Geometry check sheet. Reference: the model listing, model coordinates, mm. A direction names the side the tool comes from. Coordinates: 2 decimals unless noted, no trailing zeros. Write each loop counter-clockwise with the first axis right and the second up, starting at its lowest first coordinate (ties: lowest second). Pieces come first, ordered by that corner, then holes. Notation, with made-up numbers: M 68,38 L 112,38 A9 ccw 112,43 Z; hole C 67,20 d9. An arc over 180 degrees is marked long. Put each result on its own line as item: value. Start each with the question number.
1) Cross-section at B-B on z = -1.75. Count the separate pieces of the cut face and the enclosed holes in it, plus the area to 3 significant figures.
2) Cross-section at A-A on z = 2.5. Record the cut outline in (x, y).
3) Mould release check, pull along Y, two halves, no side actions. Record for faces 5 (the flat face through (-10.555, 0, 0)), 6 (the flat face through (10.555, 0, 0)), 7 (the flat face through (0, -11, -0.4)): released by +Y, released by -Y, zero draft, split by the parting line, or undercut.
4) Cross-section at C-C on y = 8.25. Record the cut outline in (x, z), plus the area to 3 significant figures.
5) Set-up check for faces 1 (the flat face through (-2.65, -10, -2)), 2 (the flat face through (10, 2.65, -2)), 3 (the flat face through (13.989, 0, 2)), 4 (the flat face through (1.6, -9, 1)): record each of +Z, -Z, +X, -X, +Y, -Y from which the full face is reachable in a straight line by a thin tool's end or side.
6) Scan lines: line 1 along X through (y, z) = (-8.25, 1.25); line 2 along X through (y, z) = (9.75, -0.5). Record each from-to range of solid material in increasing order.
7) Gauge pin test, flat ends, axial feed: pin 1 (2 mm diameter, centred on x = -10, z = 0.5, fed in from +Y); pin 2 (1.5 mm diameter, centred on y = -9.5, z = 3.5, fed in from -X); pin 3 (2.5 mm diameter, centred on x = -10, y = 0, fed in from -Z). Record the tip position at first contact, or that the pin passes through.
from build123d import *

# Parameters (mm, degrees)
PAD001_DEPTH    = 6.5
POCKET003_DEPTH = 5.5
PAD002_DEPTH    = 3.5
FILLET007_R     = 1
PAD009_DEPTH    = 2.4
FILLET_R        = 1
FILLET009_R     = 1
SKETCH025_W     = 5.3
SKETCH025_H     = 2
SKETCH025_W_2   = 2
SKETCH025_H_2   = 5.3
POCKET005_DEPTH = 3.1


with BuildPart() as part:
    # Sketch003 → Revolution001 (revolve)
    with BuildSketch(Plane.XZ):
        with BuildLine():
            Line((6, 3), (8, 3))
            ThreePointArc((8, 3), (7.795832, 4.795832), (7.193747, 6.5))
            Line((7.193747, 6.5), (4.570714, 6.5))
            ThreePointArc((6, 3), (5.628908, 4.890295), (4.570714, 6.5))
        make_face()
    revolve(axis=Axis((0, 0, 0), (0, 0, 1)))

    # Sketch004 (on Face1 of Revolution001) → Pad001 (new body)
    with BuildSketch(Plane(origin=(0, 0, 3), x_dir=(1, 0, 0), z_dir=(0, 0, -1))):
        with BuildLine():
            Line((4.65, -5.488852), (4.65, -13.988852))
            Line((4.65, -13.988852), (-4.65, -13.988852))
            Line((-4.65, -13.988852), (-4.65, -5.488852))
            ThreePointArc((-4.65, -5.488852), (0, -7.193747), (4.65, -5.488852))
        make_face()
        with BuildLine():
            Line((-5.488852, -4.65), (-13.988852, -4.65))
            Line((-13.988852, -4.65), (-13.988852, 4.65))
            Line((-13.988852, 4.65), (-5.488852, 4.65))
            ThreePointArc((-5.488852, 4.65), (-7.193747, 0), (-5.488852, -4.65))
        make_face()
        with BuildLine():
            Line((13.988852, -4.65), (13.988852, 4.65))
            Line((5.488852, 4.65), (13.988852, 4.65))
            ThreePointArc((5.488852, -4.65), (7.193747, 0), (5.488852, 4.65))
            Line((5.488852, -4.65), (13.988852, -4.65))
        make_face()
        with BuildLine():
            Line((-4.65, 5.488852), (-4.65, 13.988852))
            Line((-4.65, 13.988852), (4.65, 13.988852))
            Line((4.65, 13.988852), (4.65, 5.488852))
            ThreePointArc((4.65, 5.488852), (0, 7.193747), (-4.65, 5.488852))
        make_face()
    extrude(amount=PAD001_DEPTH)

    # Sketch018 (on Face24 of Pad001) → Pocket003 (cut)
    with BuildSketch(Plane(origin=(0, 0, -3.5), x_dir=(1, 0, 0), z_dir=(0, 0, -1))):
        with BuildLine():
            Line((-6.687862, 2.65), (-11.988852, 2.65))
            Line((-11.988852, 2.65), (-11.988852, -2.65))
            Line((-11.988852, -2.65), (-6.687862, -2.65))
            ThreePointArc((-6.687862, 2.65), (-7.193747, 0), (-6.687862, -2.65))
        make_face()
        with BuildLine():
            Line((-2.65, 6.687862), (-2.65, 11.988852))
            Line((-2.65, 11.988852), (2.65, 11.988852))
            Line((2.65, 11.988852), (2.65, 6.687862))
            ThreePointArc((2.65, 6.687862), (0, 7.193747), (-2.65, 6.687862))
        make_face()
        with BuildLine():
            Line((6.687862, 2.65), (11.988852, 2.65))
            Line((11.988852, 2.65), (11.988852, -2.65))
            Line((11.988852, -2.65), (6.687862, -2.65))
            ThreePointArc((6.687862, -2.65), (7.193747, 0), (6.687862, 2.65))
        make_face()
        with BuildLine():
            Line((2.65, -6.687862), (2.65, -11.988852))
            Line((2.65, -11.988852), (-2.65, -11.988852))
            Line((-2.65, -11.988852), (-2.65, -6.687862))
            ThreePointArc((-2.65, -6.687862), (0, -7.193747), (2.65, -6.687862))
        make_face()
    extrude(amount=-POCKET003_DEPTH, mode=Mode.SUBTRACT)

    # Sketch006 (on Face19 of Pocket003) → Pad002 (join)
    with BuildSketch(Plane(origin=(0, 0, 3), x_dir=(-1, 0, 0), z_dir=(0, 0, 1))):
        with BuildLine():
            Line((-13.988852, 4.65), (-5.488852, 4.65))
            ThreePointArc((-5.488852, 4.65), (-7.193747, 0), (-5.488852, -4.65))
            Line((-13.988852, -4.65), (-5.488852, -4.65))
            Line((-13.988852, -4.65), (-13.988852, 4.65))
        make_face()
        with BuildLine():
            Line((-4.65, 13.988852), (-4.65, 5.488852))
            ThreePointArc((4.65, 5.488852), (0, 7.193747), (-4.65, 5.488852))
            Line((4.65, 13.988852), (4.65, 5.488852))
            Line((-4.65, 13.988852), (4.65, 13.988852))
        make_face()
        with BuildLine():
            Line((5.488852, 4.65), (13.988852, 4.65))
            Line((13.988852, 4.65), (13.988852, -4.65))
            Line((13.988852, -4.65), (5.488852, -4.65))
            ThreePointArc((5.488852, -4.65), (7.193747, 0), (5.488852, 4.65))
        make_face()
        with BuildLine():
            Line((4.65, -5.488852), (4.65, -13.988852))
            Line((4.65, -13.988852), (-4.65, -13.988852))
            Line((-4.65, -13.988852), (-4.65, -5.488852))
            ThreePointArc((-4.65, -5.488852), (0, -7.193747), (4.65, -5.488852))
        make_face()
    extrude(amount=PAD002_DEPTH)

    # Fillet007
    fillet007_edges = [part.edges().sort_by_distance(p)[0] for p in [
        (-4.570714, 0, 6.5),
    ]]
    fillet(fillet007_edges, radius=FILLET007_R)

    # Sketch019 (on Face32 of Pad002) → Pad009 (join)
    with BuildSketch(Plane(origin=(0, 0, 2), x_dir=(1, 0, 0), z_dir=(0, 0, -1))):
        with BuildLine():
            Line((-11.988852, 2.65), (-6.687862, 2.65))
            ThreePointArc((-6.687862, 2.65), (-6.870797, 2.131231), (-7.013558, 1.6))
            Line((-7.013558, 1.6), (-10.555, 1.6))
            Line((-10.555, 1.6), (-10.555, -1.6))
            Line((-10.555, -1.6), (-7.013558, -1.6))
            ThreePointArc((-7.013558, -1.6), (-6.870797, -2.131231), (-6.687862, -2.65))
            Line((-11.988852, -2.65), (-6.687862, -2.65))
            Line((-11.988852, 2.65), (-11.988852, -2.65))
        make_face()
        with BuildLine():
            Line((-2.65, 6.687862), (-2.65, 11.988852))
            Line((-2.65, 11.988852), (2.65, 11.988852))
            Line((2.65, 11.988852), (2.65, 6.687862))
            ThreePointArc((2.65, 6.687862), (2.131231, 6.870797), (1.6, 7.013558))
            Line((1.6, 10.555), (1.6, 7.013558))
            Line((-1.6, 10.555), (1.6, 10.555))
            Line((-1.6, 7.013558), (-1.6, 10.555))
            ThreePointArc((-1.6, 7.013558), (-2.131231, 6.870797), (-2.65, 6.687862))
        make_face()
        with BuildLine():
            Line((6.687862, 2.65), (11.988852, 2.65))
            Line((11.988852, 2.65), (11.988852, -2.65))
            Line((11.988852, -2.65), (6.687862, -2.65))
            ThreePointArc((6.687862, -2.65), (6.870797, -2.131231), (7.013558, -1.6))
            Line((10.555, -1.6), (7.013558, -1.6))
            Line((10.555, 1.6), (10.555, -1.6))
            Line((7.013558, 1.6), (10.555, 1.6))
            ThreePointArc((7.013558, 1.6), (6.870797, 2.131231), (6.687862, 2.65))
        make_face()
        with BuildLine():
            Line((2.65, -11.988852), (-2.65, -11.988852))
            Line((-2.65, -11.988852), (-2.65, -6.687862))
            ThreePointArc((-2.65, -6.687862), (-2.131231, -6.870797), (-1.6, -7.013558))
            Line((-1.6, -7.013558), (-1.6, -10.555))
            Line((-1.6, -10.555), (1.6, -10.555))
            Line((1.6, -10.555), (1.6, -7.013558))
            ThreePointArc((1.6, -7.013558), (2.131231, -6.870797), (2.65, -6.687862))
            Line((2.65, -6.687862), (2.65, -11.988852))
        make_face()
    extrude(amount=PAD009_DEPTH)

    # Fillet
    fillet_edges = [part.edges().sort_by_distance(p)[0] for p in [
        (10.555, 0, 2),
        (0, -10.555, 2),
        (-10.555, 0, 2),
        (0, 10.555, 2),
    ]]
    fillet(fillet_edges, radius=FILLET_R)

    # Fillet009
    fillet009_edges = [part.edges().sort_by_distance(p)[0] for p in [
        (13.988852, 0, 6.5),
        (0, 13.988852, 6.5),
        (-13.988852, 0, 6.5),
        (0, -13.988852, 6.5),
    ]]
    fillet(fillet009_edges, radius=FILLET009_R)

    # Sketch025 (on Face48 of Fillet009) → Pocket005 (cut)
    with BuildSketch(Plane(origin=(0, 0, -3.5), x_dir=(1, 0, 0), z_dir=(0, 0, -1))):
        with Locations((0, -12.988852)):
            Rectangle(SKETCH025_W, SKETCH025_H)
        with Locations((12.988852, 0)):
            Rectangle(SKETCH025_W_2, SKETCH025_H_2)
        with Locations((0, 12.988852)):
            Rectangle(SKETCH025_W, SKETCH025_H)
        with Locations((-12.988852, 0)):
            Rectangle(SKETCH025_W_2, SKETCH025_H_2)
    extrude(amount=-POCKET005_DEPTH, mode=Mode.SUBTRACT)


solid = part.part
Answer key:
1. separate pieces: 8
1. enclosed holes: 0
1. area: 125 mm²
2. outline: M -13.99,-4.65 L -5.49,-4.65 A7.19 cw -5.49,4.65 L -13.99,4.65 Z; M -4.65,-13.99 L 4.65,-13.99 L 4.65,-5.49 A7.19 cw -4.65,-5.49 Z; M -4.65,5.49 A7.19 cw 4.65,5.49 L 4.65,13.99 L -4.65,13.99 Z; M 5.49,-4.65 L 13.99,-4.65 L 13.99,4.65 L 5.49,4.65 A7.19 cw Z
3. face 5: undercut
3. face 6: undercut
3. face 7: zero draft
4. outline: M -4.65,-3.5 L -2.65,-3.5 L -2.65,-0.4 L -1.6,-0.4 L -1.6,2 L 1.6,2 L 1.6,-0.4 L 2.65,-0.4 L 2.65,-3.5 L 4.65,-3.5 L 4.65,6.5 L -4.65,6.5 Z
4. area: 68.9 mm²
5. face 1: -Z, +Y, -Y
5. face 2: -Z, +X, -X
5. face 3: +Z, -Z, +X, +Y, -Y
5. face 4: -Z
6. line 1: x = -4.65 to -1.6, 1.6 to 4.65
6. line 2: x = -4.65 to -2.65, 2.65 to 4.65
7. pin 1: stops at y = 4.65
7. pin 2: stops at x = -4.65
7. pin 3: stops at z = -0.4
